Build history of the part. All positions in model axes, mm. Round coordinates to 2 decimals unless told otherwise and drop trailing zeros. Loops run counter-clockwise (first coordinate to the right, second up) from the corner with the lowest first, then second, coordinate; pieces in that order, holes last. Notation, with made-up numbers: (51.5, 17) - (75.5, 17) arc R16 ccw to (75.5, 28) - close; hole circle Ø10 at (77, 55.5). An arc over 180 degrees is marked (long way). One line per question, with ' | ' between items. Start each with the question number.
from build123d import *

# Parameters (mm, degrees)
F1_DEPTH = 208.333333
F2_R     = 3.25
F3_DEPTH = 10
F4_R     = 3.25
F5_DEPTH = 10


with BuildPart() as f1:
    # F0 (on Front) → F1 (new body)
    with BuildSketch(Plane.XZ):
        Polygon((0, 0), (8.854167, 0), (17.708333, 0), (17.708333, 11.354167), (16.354167, 12.604167), (16.354167, 21.354167), (17.708333, 22.604167), (17.708333, 31.25), (8.854167, 31.25), (0, 31.25), (0, 22.604167), (1.354167, 21.354167), (1.354167, 12.604167), (0, 11.354167), align=None)
    extrude(amount=F1_DEPTH)

    # F2 (on face) → F3 (cut)
    with BuildSketch(Plane.XZ.offset(208.333333)):
        with Locations((8.854167, 6)):
            Circle(F2_R)
        with Locations((8.854167, 25.25)):
            Circle(F2_R)
    extrude(amount=-F3_DEPTH, mode=Mode.SUBTRACT)

    # F4 (on face) → F5 (cut)
    with BuildSketch(Plane(origin=(0, 0, 0), x_dir=(-1, 0, 0), z_dir=(0, 1, 0))):
        with Locations((-8.854167, 6)):
            Circle(F4_R)
        with Locations((-8.854167, 25.25)):
            Circle(F4_R)
    extrude(amount=-F5_DEPTH, mode=Mode.SUBTRACT)


solid = f1.part
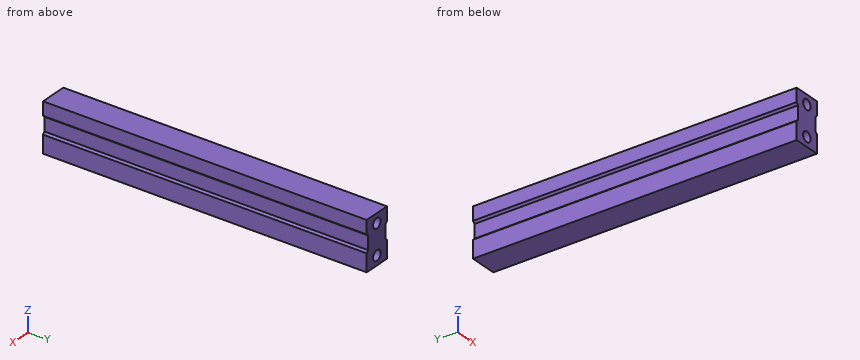
1) Wall check: line 1 (Y direction, x = 11.75, z = 5.5); line 2 (X direction, y = -55.5, z = 18); line 3 (Z direction, x = 16.5, y = -162). Give the ranges that are in metal, low to high. Write a range as [from, to].
2) Saw through at D-D on z = 16.5. Write the cut outline in (x, y).
3) Saw through at C-C on x = 9. Write the cut outline in (y, z).
4) Drop flat-ended pins along their axis: pin 1 (6 mm diameter, centred on x = 8.85, z = 25.25, fed in from -Y); pin 2 (4.5 mm diameter, centred on y = -119.5, z = 16.5, fed in from -X); pin 3 (2 mm diameter, centred on x = 10.5, z = 5, fed in from +Y). Give the stop position or say it passes through.
5) Saw through at B-B on y = -160. Write the cut outline in (x, z).
6) Saw through at A-A on z = 25.25. Write the cut outline in (x, y).
Answer key:
1) line 1: [-198.33, -10] | line 2: [1.35, 16.35] | line 3: [0, 12.47], [21.49, 31.25]
2) outline: (1.35, -208.33) - (16.35, -208.33) - (16.35, 0) - (1.35, 0) - close
3) outline: (-208.33, 0) - (0, 0) - (0, 2.75) - (-10, 2.75) - (-10, 9.25) - (0, 9.25) - (0, 22) - (-10, 22) - (-10, 28.5) - (0, 28.5) - (0, 31.25) - (-208.33, 31.25) - (-208.33, 28.5) - (-198.33, 28.5) - (-198.33, 22) - (-208.33, 22) - (-208.33, 9.25) - (-198.33, 9.25) - (-198.33, 2.75) - (-208.33, 2.75) - close
4) pin 1: y = -198.33 | pin 2: x = 1.35 | pin 3: y = -10
5) outline: (0, 0) - (17.71, 0) - (17.71, 11.35) - (16.35, 12.6) - (16.35, 21.35) - (17.71, 22.6) - (17.71, 31.25) - (0, 31.25) - (0, 22.6) - (1.35, 21.35) - (1.35, 12.6) - (0, 11.35) - close
6) outline: (0, -208.33) - (5.6, -208.33) - (5.6, -198.33) - (12.1, -198.33) - (12.1, -208.33) - (17.71, -208.33) - (17.71, 0) - (12.1, 0) - (12.1, -10) - (5.6, -10) - (5.6, 0) - (0, 0) - close
